Geometry check sheet. Reference: drawing and pictorial views, mm from the part's lowest x, y, z. Round coordinates to 2 decimals unless told otherwise and drop trailing zeros. Write each loop counter-clockwise with the first axis right and the second up, starting at its lowest first coordinate (ties: lowest second). Pieces come first, ordered by that corner, then holes. Notation, with made-up numbers: M -2,66 L 17,66 A14 cw 17,93 Z; hole C -28,87.25 d11. An arc over 180 degrees is marked long. Answer in a Markdown table with one row per item. Add a question column.
1. Material ranges on probe 1 along Z at (x, y) = (0.95, 85); probe 2 along Y at (x, z) = (2, 18); probe 3 along Y at (x, z) = (1.5, 90), recorded low to high.
2. Sectioned sample at B-B on z = 90. Record the cut outline in (x, y).
3. Sectioned sample at A-A on y = 45. Record the cut outline in (x, z), plus the area to 3 significant figures.
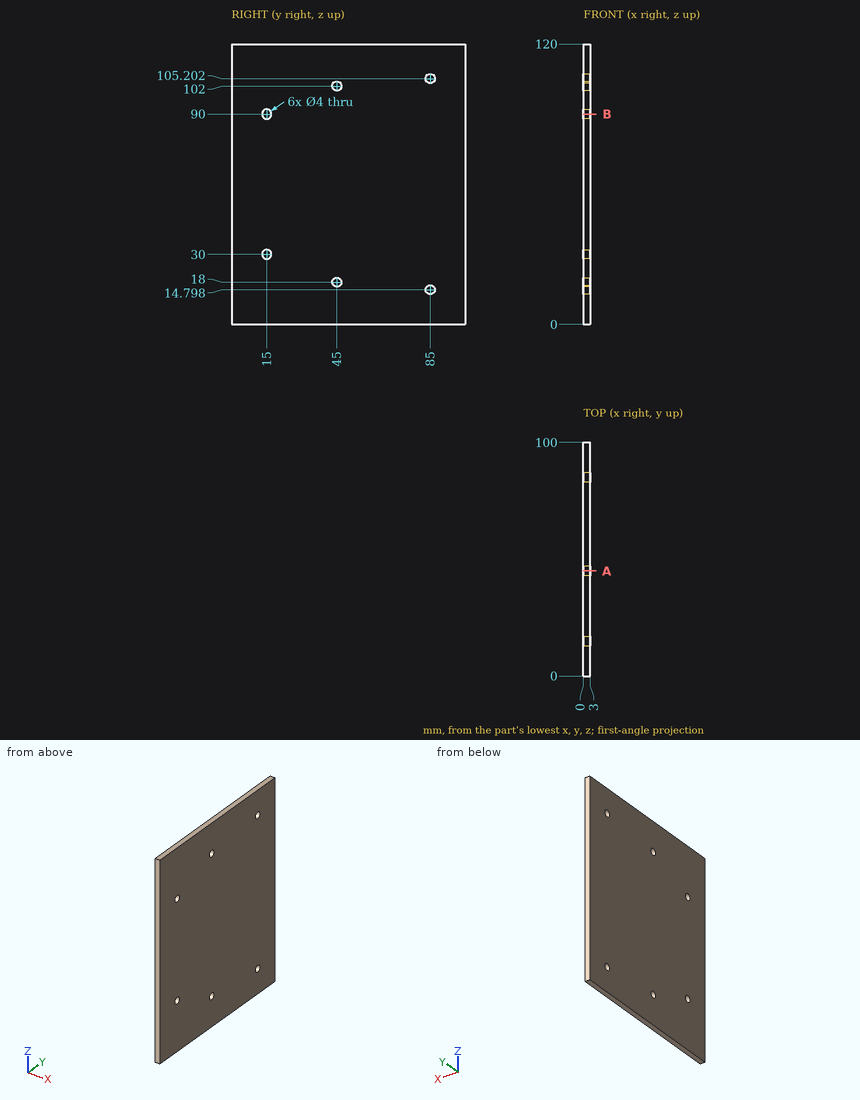
Geometry check:
| question | item | result |
|---|---|---|
| 1 | probe 1 | z = 0 to 12.8, 16.8 to 103.2, 107.2 to 120 |
| 1 | probe 2 | y = 0 to 43, 47 to 100 |
| 1 | probe 3 | y = 0 to 13, 17 to 100 |
| 2 | outline | M 0,0 L 3,0 L 3,13 L 0,13 Z; M 0,17 L 3,17 L 3,100 L 0,100 Z |
| 3 | outline | M 0,0 L 3,0 L 3,16 L 0,16 Z; M 0,20 L 3,20 L 3,100 L 0,100 Z; M 0,104 L 3,104 L 3,120 L 0,120 Z |
| 3 | area | 336 mm2 |
